Geometry check sheet. Reference: the model listing, model coordinates, mm. Face numbers are marked on the shaded views. A direction names the side the tool comes from. Coordinates: 2 decimals unless noted, no trailing zeros. Write each loop counter-clockwise with the first axis right and the second up, starting at its lowest first coordinate (ties: lowest second). Pieces come first, ordered by that corner, then holes. Notation, with made-up numbers: (17.5, -35) -> (23.5, -35) arc R26 ccw to (23.5, -17) -> close; hole circle Ø2 at (43, -28.5). An arc over 180 degrees is marked (long way). One line per question, with ' | ' between items.
from build123d import *

# Parameters (mm, degrees)
BOSS_EXTRUDE1_DEPTH = 3
BOSS_EXTRUDE2_START = -6.36
BOSS_EXTRUDE2_DEPTH = 3
BOSS_EXTRUDE3_START = -3
BOSS_EXTRUDE3_DEPTH = 12.36
CUT_EXTRUDE1_DEPTH  = 1


with BuildPart() as part:
    # Sketch1 → Boss-Extrude1 (new body)
    with BuildSketch(Plane.XZ.offset(32.361588827)):
        with BuildLine():
            Line((-28.868957331, -307.014773368), (-29.868957331, -301.096085324))
            ThreePointArc((-29.868957331, -301.096085324), (-47.432277428, -302.971340874), (-65.04446736, -301.630608989))
            Line((-65.04446736, -301.630608989), (-65.981716568, -307.557257918))
            ThreePointArc((-65.981716568, -307.557257918), (-47.400699357, -308.971536481), (-28.868957331, -307.014773368))
        make_face()
    extrude(amount=BOSS_EXTRUDE1_DEPTH)



with BuildPart() as body_2:
    # Sketch1<2> → Boss-Extrude2 (new body)
    with BuildSketch(Plane.XZ.offset(32.361588827).offset(BOSS_EXTRUDE2_START)):
        with BuildLine():
            Line((-28.868957331, -307.014773368), (-29.868957331, -301.096085324))
            ThreePointArc((-29.868957331, -301.096085324), (-47.432277428, -302.971340874), (-65.04446736, -301.630608989))
            Line((-65.04446736, -301.630608989), (-65.981716568, -307.557257918))
            ThreePointArc((-65.981716568, -307.557257918), (-47.400699357, -308.971536481), (-28.868957331, -307.014773368))
        make_face()
    extrude(amount=-BOSS_EXTRUDE2_DEPTH)


with BuildPart() as part_1:
    add(part.part)

    add(body_2.part)  # Boss-Extrude3 merges body 2
    # Sketch2 → Boss-Extrude3 (add)
    with BuildSketch(Plane(origin=(0, -26.001588827, 0), x_dir=(-1, 0, 0), z_dir=(0, -1, 0)).offset(BOSS_EXTRUDE3_START)):
        with BuildLine():
            ThreePointArc((65.981716568, 307.557257918), (47.400699357, 308.971536481), (28.868957331, 307.014773368))
            ThreePointArc((28.868957331, 307.014773368), (47.324504287, 314.184236637), (65.981716568, 307.557257918))
        make_face()
    extrude(amount=BOSS_EXTRUDE3_DEPTH)

    # Sketch4 → Cut-Extrude1 (cut)
    with BuildSketch(Plane(origin=(0, -23.001588827, 0), x_dir=(1, 0, 0), z_dir=(0, 1, 0))):
        with BuildLine():
            ThreePointArc((-63.492663367, 309.420035692), (-64.18989584, 308.940344318), (-64.87253134, 308.44009867))
            Line((-64.87253134, 308.44009867), (-29.951864875, 307.929656373))
            ThreePointArc((-29.951864875, 307.929656373), (-30.619587474, 308.449640474), (-31.302501574, 308.949505723))
            Line((-31.302501574, 308.949505723), (-63.492663367, 309.420035692))
        make_face()
        with BuildLine():
            ThreePointArc((-60.073849839, 311.370275869), (-61.00439253, 310.900603204), (-61.917080112, 310.397111905))
            Line((-61.917080112, 310.397111905), (-32.848853555, 309.972215882))
            ThreePointArc((-32.848853555, 309.972215882), (-33.746435087, 310.502168243), (-34.662852555, 310.99883829))
            Line((-34.662852555, 310.99883829), (-60.073849839, 311.370275869))
        make_face()
        with BuildLine():
            ThreePointArc((-54.80969362, 313.293542306), (-56.329988828, 312.857479245), (-57.823662491, 312.33749126))
            Line((-57.823662491, 312.33749126), (-36.88380863, 312.03140927))
            ThreePointArc((-36.88380863, 312.03140927), (-38.361645858, 312.594832417), (-39.868546228, 313.075144596))
            Line((-39.868546228, 313.075144596), (-54.80969362, 313.293542306))
        make_face()
    cut_extrude1 = extrude(amount=-CUT_EXTRUDE1_DEPTH, mode=Mode.SUBTRACT)

    # Mirror1: Cut-Extrude1 across plane
    add(cut_extrude1.mirror(Plane(origin=(0, -29.181588827, 0), x_dir=(0, 0, 1), z_dir=(0, -1, 0))), mode=Mode.SUBTRACT)


solid = part_1.part
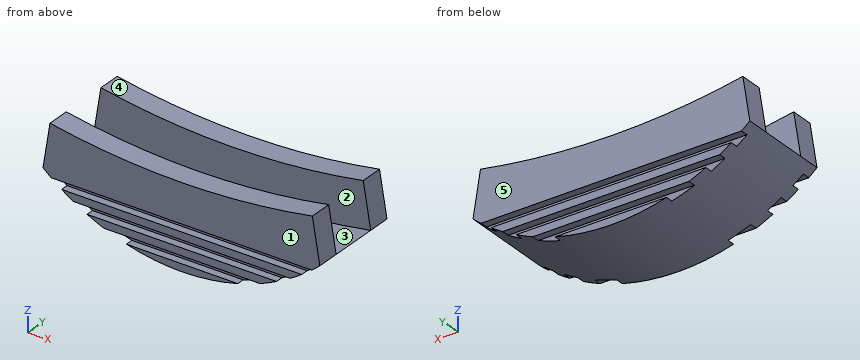
1. Mould release check, pull along Y, two halves, no side actions. Record for the marked faces 3, 4 and 5: released by +Y, released by -Y, zero draft, split by the parting line, or undercut.
Worked answers:
face 3: undercut | face 4: zero draft | face 5: released by +Y
2. Cross-section at D-D on y = -25. Record the boundary of the cut face in (x, z), and give its area (3 significant figures).
Worked answers:
outline: (-65.98, -307.56) arc R28.41 ccw to (-28.87, -307.01) -> (-29.87, -301.1) arc R97 cw to (-65.04, -301.63) -> close | area: 352 mm²
3. Tool access check on the marked faces 1 and 2. Record the directions out of +Z, -Z, +X, -X, +Y, -Y that give a thin tool (end or side, any length) a straight path to the whole face; none if there is none.
Worked answers:
face 1: +Z, -Z, +X, -X, -Y | face 2: +Z
4. Go/stop test with flat-tipped pins: P1, Ø0.7, axis at x = -40.5, z = -310.5, coming from the -Y side; P2, Ø1, axis at x = -42.5, y = -31.5, coming from the -Z side; P3, Ø2, axis at y = -30, z = -311, coming from the +X side. Record where each tip stops, or that it passes through.
Worked answers:
P1: y = -34.36 | P2: z = -313.79 | P3: x = -32.89
5. Material ranges on line 1 (Y direction, x = -39, z = -303.75); line 2 (Z direction, x = -56, y = -23.75); line 3 (Y direction, x = -45, z = -312.5), recorded low to high. Write a range as from..to.
Worked answers:
line 1: -35.36..-32.36, -26..-23 | line 2: -312.31..-311.31, -310.31..-309.31, -308.31..-302.72 | line 3: -34.36..-24
6. Cross-section at B-B on z = -302.5. Record the boundary of the cut face in (x, y).
Worked answers:
outline: (-65.18, -35.36) -> (-58.57, -35.36) -> (-58.57, -32.36) -> (-65.18, -32.36) -> close; (-65.18, -26) -> (-58.57, -26) -> (-58.57, -23) -> (-65.18, -23) -> close; (-39.24, -35.36) -> (-29.63, -35.36) -> (-29.63, -32.36) -> (-39.24, -32.36) -> close; (-39.24, -26) -> (-29.63, -26) -> (-29.63, -23) -> (-39.24, -23) -> close
7. Cross-section at A-A on z = -305. Record the boundary of the cut face in (x, y), and give its area (3 significant figures).
Worked answers:
outline: (-65.58, -35.36) -> (-29.21, -35.36) -> (-29.21, -32.36) -> (-65.58, -32.36) -> close; (-65.58, -26) -> (-29.21, -26) -> (-29.21, -23) -> (-65.58, -23) -> close | area: 218 mm²
